Read the model definition and answer for the solid it produces. Units are mm, in the model's axes. Coordinates: 2 decimals unless noted, no trailing zeros. Write each loop counter-clockwise with the first axis right and the second up, starting at its lowest first coordinate (ties: lowest second). Pieces come first, ordered by that corner, then holes. Notation, with made-up numbers: M 24.5,-32.75 L 77.5,-32.75 A20 cw 77.5,-12.75 Z; hole C 85,-19.5 d10. An arc over 180 degrees is marked long. Write item = value, one per line.
from build123d import *

# Parameters (mm, degrees)
SKETCH1_W           = 500
SKETCH1_H           = 400
BOSS_EXTRUDE1_DEPTH = 10
SKETCH2_W           = 400
SKETCH2_H           = 50
BOSS_EXTRUDE2_DEPTH = 10
SKETCH3_R           = 5
BOSS_EXTRUDE5_DEPTH = 50


with BuildPart() as part:
    # Sketch1 → Boss-Extrude1 (new body)
    with BuildSketch(Plane(origin=(0, 0, 0), x_dir=(1, 0, 0), z_dir=(0, 1, 0))):
        Rectangle(SKETCH1_W, SKETCH1_H)
    extrude(amount=BOSS_EXTRUDE1_DEPTH)

    # Sketch2 → Boss-Extrude2 (add)
    with BuildSketch(Plane(origin=(0, 10, 0), x_dir=(1, 0, 0), z_dir=(0, 1, 0))):
        with Locations((0, 225)):
            Rectangle(SKETCH2_W, SKETCH2_H)
    extrude(amount=-BOSS_EXTRUDE2_DEPTH)

    # Sketch3 → Boss-Extrude5 (add)
    with BuildSketch(Plane.ZY.offset(200)):
        with Locations(Location((-240, 5, 0), (0, 0, 270))):
            Circle(SKETCH3_R)
    boss_extrude5 = extrude(amount=BOSS_EXTRUDE5_DEPTH)

    # Mirror1: Boss-Extrude5 across plane
    add(boss_extrude5.mirror(Plane(origin=(0, 0, 0), x_dir=(0, 0, 1), z_dir=(1, 0, 0))))


solid = part.part
Item 1: Find section A-A (y = 5). Determine the outline of the cut face in (x, z), and give its area (3 significant figures).
Worked answers:
outline = M -250,-245 L -200,-245 L -200,-250 L 200,-250 L 200,-245 L 250,-245 L 250,-235 L 200,-235 L 200,-200 L 250,-200 L 250,200 L -250,200 L -250,-200 L -200,-200 L -200,-235 L -250,-235 Z
area = 221,000 mm²
Item 2: Consider line 1 along Z through (x, y) = (-207, 4.25); line 2 along Z through (x, y) = (201.5, 7.25); line 3 along X through (y, z) = (8.75, -227). Determine where each line is inside the solid, lowest interval first. Write a range as from..to.
Worked answers:
line_1 = -244.94..-235.06, -200..200
line_2 = -244.47..-235.53, -200..200
line_3 = -200..200
Item 3: Flat-ended cylindrical pins translate along their axes: pin 1 (3 mm diameter, centred on x = 229, y = 2.5, fed in from -Z); pin 2 (5 mm diameter, centred on y = 4.5, z = -215, fed in from -X); pin 3 (3 mm diameter, centred on y = 5, z = -222, fed in from +X). Find the tip coordinate at first contact, or state that the pin passes through.
Worked answers:
pin_1 = -244.9
pin_2 = -200
pin_3 = 200
